```python
from build123d import *

# Parameters (mm, degrees)
SKETCH2_W               = 508
SKETCH2_H               = 101.6
BOSS_EXTRUDE2_DEPTH     = 965.2
SKETCH3_R               = 25.4
SKETCH3_W               = 25.4
SKETCH3_H               = 25.4
CUT_EXTRUDE1_DEPTH      = 50.8
CUT_EXTRUDE2_DEPTH      = 1096.444019565
CUT_EXTRUDE2_DEPTH_BACK = 1096.444019565
FILLET1_R               = 17.78
FILLET6_R               = 50.8
SKETCH5_R               = 76.2
BOSS_EXTRUDE3_DEPTH     = 50.8
FILLET2_R               = 12.7
CHAMFER1_SIZE           = 7.46
CHAMFER1_SIZE2          = 8.890481801


with BuildPart() as part:
    # Sketch2 → Boss-Extrude2 (new body)
    with BuildSketch(Plane.XY):
        with Locations((254, 50.8)):
            Rectangle(SKETCH2_W, SKETCH2_H)
    extrude(amount=BOSS_EXTRUDE2_DEPTH)

    # Sketch3 → Cut-Extrude1 (cut)
    with BuildSketch(Plane(origin=(0, 0, 0), x_dir=(-1, 0, 0), z_dir=(0, -1, 0))):
        with Locations(Location((-50.8, -762, 0), (0, 0, 90))):
            Circle(SKETCH3_R)
        with Locations(Location((-457.2, -762, 0), (0, 0, 90))):
            Circle(SKETCH3_R)
        with Locations((-457.2, -215.9)):
            Rectangle(SKETCH3_W, SKETCH3_H)
        with Locations((-50.8, -215.9)):
            Rectangle(SKETCH3_W, SKETCH3_H)
    extrude(amount=-CUT_EXTRUDE1_DEPTH, mode=Mode.SUBTRACT)

    # Sketch4 → Cut-Extrude2 (cut, two sides: drawn at the far end of the back side and taken through both)
    with BuildSketch(Plane.XZ.offset(-CUT_EXTRUDE2_DEPTH_BACK)):
        Polygon((101.6, 965.2), (406.4, 965.2), (508, 965.2), (508, 838.2), (406.4, 838.2), (406.4, 584.2), (101.6, 584.2), (101.6, 838.2), (0, 838.2), (0, 965.2), align=None)
        Polygon((101.6, 381), (406.4, 381), (406.4, 152.4), (508, 152.4), (508, 0), (406.4, 0), (101.6, 0), (0, 0), (0, 152.4), (101.6, 152.4), align=None)
    extrude(amount=CUT_EXTRUDE2_DEPTH + CUT_EXTRUDE2_DEPTH_BACK, mode=Mode.SUBTRACT)

    # Fillet1
    fillet1_edges = [part.edges().sort_by_distance(p)[0] for p in [
        (0, 101.6, 495.3),
        (508, 101.6, 495.3),
        (406.4, 101.6, 711.2),
        (406.4, 50.8, 584.2),
        (254, 101.6, 584.2),
        (101.6, 50.8, 584.2),
        (101.6, 101.6, 711.2),
        (457.2, 101.6, 838.2),
        (50.8, 101.6, 838.2),
        (101.6, 50.8, 152.4),
        (101.6, 101.6, 266.7),
        (101.6, 50.8, 381),
        (254, 101.6, 381),
        (406.4, 50.8, 381),
        (406.4, 101.6, 266.7),
        (406.4, 50.8, 152.4),
        (457.2, 101.6, 152.4),
        (0, 50.8, 152.4),
        (50.8, 101.6, 152.4),
        (508, 50.8, 152.4),
    ]]
    fillet(fillet1_edges, radius=FILLET1_R)

    # Fillet6
    # the kernel refuses this fillet: 50.8 mm, written as the material it takes off along each edge
    with BuildSketch(Plane(origin=(50.8, 101.6, 787.4), x_dir=(-1, 0, 0), z_dir=(0, 0, -1))) as fillet6_piece_1:
        with BuildLine():
            CenterArc((33.02, -17.78), 17.78, 0, 90)
            Line((50.8, -17.78), (50.8, 0))
            Line((50.8, 0), (33.02, 0))
        make_face()
    revolve(axis=Axis((50.8, 101.6, 787.4), (0, 1, 0)), revolution_arc=90, mode=Mode.SUBTRACT)
    with BuildSketch(Plane(origin=(50.8, 101.6, 787.4), x_dir=(0, 0, 1), z_dir=(-1, 0, 0))) as fillet6_piece_2:
        with BuildLine():
            CenterArc((33.02, -17.78), 17.78, 0, 90)
            Line((50.8, -17.78), (50.8, 0))
            Line((50.8, 0), (33.02, 0))
        make_face()
    revolve(axis=Axis((50.8, 101.6, 787.4), (0, 1, 0)), revolution_arc=90, mode=Mode.SUBTRACT)
    with BuildSketch(Plane(origin=(457.2, 101.6, 787.4), x_dir=(-1, 0, 0), z_dir=(0, 0, -1))) as fillet6_piece_3:
        with BuildLine():
            CenterArc((33.02, -17.78), 17.78, 0, 90)
            Line((50.8, -17.78), (50.8, 0))
            Line((50.8, 0), (33.02, 0))
        make_face()
    revolve(axis=Axis((457.2, 101.6, 787.4), (0, 1, 0)), revolution_arc=90, mode=Mode.SUBTRACT)
    with BuildSketch(Plane(origin=(457.2, 101.6, 787.4), x_dir=(0, 0, 1), z_dir=(-1, 0, 0))) as fillet6_piece_4:
        with BuildLine():
            CenterArc((33.02, -17.78), 17.78, 0, 90)
            Line((50.8, -17.78), (50.8, 0))
            Line((50.8, 0), (33.02, 0))
        make_face()
    revolve(axis=Axis((457.2, 101.6, 787.4), (0, 1, 0)), revolution_arc=90, mode=Mode.SUBTRACT)
    with BuildSketch(Plane(origin=(508, -127, 838.2), x_dir=(-1, 0, 0), z_dir=(0, 1, 0)), Plane(origin=(406.4, -127, 838.2), x_dir=(0, 0, -1), z_dir=(0, 1, 0))) as fillet6_piece_5:
        with BuildLine():
            CenterArc((FILLET6_R, -FILLET6_R), FILLET6_R, 90, 90)
            Line((0, -FILLET6_R), (0, 0))
            Line((0, 0), (FILLET6_R, 0))
        make_face()
    extrude(amount=228.6, mode=Mode.SUBTRACT)
    with BuildSketch(Plane(origin=(101.6, 101.6, 838.2), x_dir=(-1, 0, 0), z_dir=(0, -1, 0)), Plane(origin=(0, 101.6, 838.2), x_dir=(0, 0, -1), z_dir=(0, -1, 0))) as fillet6_piece_6:
        with BuildLine():
            CenterArc((FILLET6_R, FILLET6_R), FILLET6_R, 180, 90)
            Line((0, FILLET6_R), (0, 0))
            Line((0, 0), (FILLET6_R, 0))
        make_face()
    extrude(amount=228.6, mode=Mode.SUBTRACT)

    # Sketch5 → Boss-Extrude3 (add)
    with BuildSketch(Plane(origin=(0, 101.6, 0), x_dir=(1, 0, 0), z_dir=(0, 1, 0))):
        with Locations((254, -482.6)):
            Circle(SKETCH5_R)
    extrude(amount=BOSS_EXTRUDE3_DEPTH)

    # Fillet2
    fillet2_edges = [part.edges().sort_by_distance(p)[0] for p in [
        (177.8, 101.6, 482.6),
    ]]
    fillet(fillet2_edges, radius=FILLET2_R)

    # Chamfer1
    chamfer1_edges = [part.edges().sort_by_distance(p)[0] for p in [
        (177.8, 152.4, 482.6),
    ]]
    chamfer1_side = [part.faces().sort_by_distance(p)[0] for p in [
        (177.8, 133.057233691, 482.6),
    ]]
    chamfer(chamfer1_edges, length=CHAMFER1_SIZE, length2=CHAMFER1_SIZE2, reference=chamfer1_side[0])


solid = part.part
```
The model under review builds one solid part; all positions refer to its coordinate system, in mm. A direction names the side the tool comes from. Coordinates: 2 decimals unless noted, no trailing zeros. Order: outer loops, then holes, each group sorted by start corner. A loop starts at its lowest first (then second) coordinate and runs counter-clockwise, first axis right, second up. Notation, with made-up numbers: (63, 87.5) -> (69, 87.5) arc R20 cw to (69, 96.5) -> close; hole circle Ø10 at (41, -11). An arc over 180 degrees is marked (long way). Answer in a Markdown table with one row per item. Add a question column.
Item 1: We need section A-A on z = 622.5. Write out the cut boundary in (x, y).
Item 2: We need section D-D on z = 482.6. Write out the cut boundary in (x, y), plus the area to 3 significant figures.
Item 3: Machinability: for faces 1 (the flat face through (250, 0, 490)), 2 (the flat face through (406.4, 42, 268)), 3 (the cylindrical face through (106.947, 41.323, 589.27)), 4 (the flat face through (508, 41, 474)), 5 (the cylindrical face through (255.885, 96.53, 386.347)), which of the approach directions +Z, -Z, +X, -X, +Y, -Y give a long, thin tool a straight path to every point of the face, cutting with its end or side? Answer none if there is none.
Item 4: To check wall thickness, follow probe 1 along X at (y, z) = (41, 762); probe 2 along Z at (x, y) = (457, 15); probe 3 along X at (y, z) = (57, 609). State the ranges of each line that lie inside material, in increasing order.
Item 5: We need section C-C on y = 34. Give the number of separate pieces and of enclosed holes in the cut face, plus the area to 3 significant figures.
Item 6: Clearance check with flat-ended pins moving along their axes: pin 1 (12 mm diameter, centred on x = 234.5, y = 111, fed in from -Z); pin 2 (15 mm diameter, centred on x = 45.5, z = 756.5, fed in from -Y); pin 3 (4 mm diameter, centred on x = 57, y = 101.5, fed in from +Z). State where each tip first meets the part, or that it passes through.
Item 7: We need section B-B on x = 50.8. Write out the cut boundary in (y, z).
Item 8: Mouldability with a two-part tool opening along Z and no side actions: class faces 6 (the cylindrical face through (401.33, 41.323, 589.547)), 7 (the flat face through (101.6, 42, 265)), 8 (the flat face through (444.5, 25, 216)), 9 (the flat face through (457, 25, 203.2)) as +Z half, -Z half, draft (parallel to the pull), parting line (faces both ways), or undercut.
Final values:
| question | item | result |
|---|---|---|
| 1 | outline | (0, 0) -> (101.6, 0) -> (101.6, 83.82) arc R17.78 ccw to (83.82, 101.6) -> (17.78, 101.6) arc R17.78 ccw to (0, 83.82) -> close; (406.4, 0) -> (508, 0) -> (508, 83.82) arc R17.78 ccw to (490.22, 101.6) -> (424.18, 101.6) arc R17.78 ccw to (406.4, 83.82) -> close |
| 2 | outline | (0, 0) -> (508, 0) -> (508, 83.82) arc R17.78 ccw to (490.22, 101.6) -> (342.9, 101.6) arc R12.7 cw to (330.2, 114.3) -> (330.2, 144.94) -> (321.31, 152.4) -> (186.69, 152.4) -> (177.8, 144.94) -> (177.8, 114.3) arc R12.7 cw to (165.1, 101.6) -> (17.78, 101.6) arc R17.78 ccw to (0, 83.82) -> close |
| 2 | area | 59,200 mm2 |
| 3 | face 1 | +Z, -Z, +X, -X, -Y |
| 3 | face 2 | -Z, +Y, -Y |
| 3 | face 3 | +Z, +Y, -Y |
| 3 | face 4 | +Z, -Z, +X, +Y, -Y |
| 3 | face 5 | -Z, +Y |
| 4 | probe 1 | x = 0 to 25.4, 76.2 to 101.6, 406.4 to 431.8, 482.6 to 508 |
| 4 | probe 2 | z = 152.4 to 203.2, 228.6 to 736.6, 787.4 to 838.2 |
| 4 | probe 3 | x = 0 to 101.6, 406.4 to 508 |
| 5 | separate pieces | 1 |
| 5 | enclosed holes | 4 |
| 5 | area | 194,000 mm2 |
| 6 | pin 1 | stops at z = 404.73 |
| 6 | pin 2 | stops at y = 50.8 |
| 6 | pin 3 | stops at z = 828.35 |
| 7 | outline | (0, 152.4) -> (83.82, 152.4) arc R17.78 ccw to (101.6, 170.18) -> (101.6, 820.42) arc R17.78 ccw to (83.82, 838.2) -> (0, 838.2) -> (0, 787.4) -> (50.8, 787.4) -> (50.8, 736.6) -> (0, 736.6) -> (0, 228.6) -> (50.8, 228.6) -> (50.8, 203.2) -> (0, 203.2) -> close |
| 8 | face 6 | +Z half |
| 8 | face 7 | draft |
| 8 | face 8 | undercut |
| 8 | face 9 | undercut |
